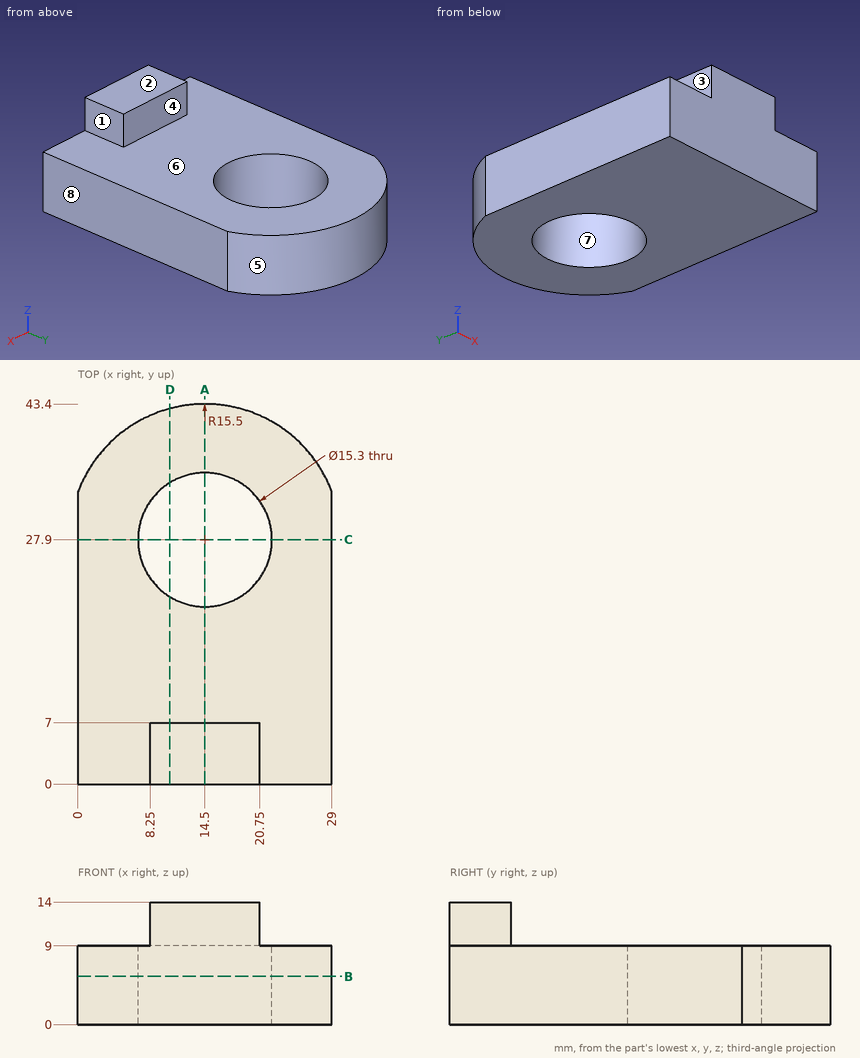
Design review of the part shown in the three views and the two pictorial views. Dimensions are in mm from the part's minimum x, y and z. A direction names the side the tool comes from. Round coordinates to 2 decimals unless told otherwise and drop trailing zeros. Write each loop counter-clockwise with the first axis right and the second up, starting at its lowest first coordinate (ties: lowest second). Pieces come first, ordered by that corner, then holes. Notation, with made-up numbers: (-28, 86.5) -> (18, 86.5) arc R28 cw to (18, 125.5) -> close; hole circle Ø10 at (84.5, 33). An arc over 180 degrees is marked (long way). One line per question, with ' | ' between items. Start each with the question number.
1) Add section D-D (x = 10.5). Write out the cut boundary in (y, z), and give its area (3 significant figures).
2) Mouldability with a two-part tool opening along X and no side actions: class the marked faces 6, 7 and 8 as +X half, -X half, draft (parallel to the pull), parting line (faces both ways), or undercut.
3) Add section C-C (y = 27.9). Write out the cut boundary in (x, z).
4) For pin 1 Ø8.5 at (x, y) = (19.5, 24.5) entering from +Z; pin 2 Ø5.5 at (x, z) = (17.5, 12) entering from +Y; pin 3 Ø1.5 at (y, z) = (3.5, 11.5) entering from -X, all flat-tipped, find the tip position at first contact; note any pin that passes through.
5) Add section A-A (x = 14.5). Write out the cut boundary in (y, z), and give its area (3 significant figures).
6) Add section B-B (z = 5.5). Write out the cut boundary in (x, y), and give its area (3 significant figures).
7) Machinability: for the marked faces 1, 2, 3, 4 and 5, which of the approach directions +Z, -Z, +X, -X, +Y, -Y give a long, thin tool a straight path to every point of the face, cutting with its end or side? Answer none if there is none.
8) Wall thickness on line 1 along Y through (x, z) = (14.5, 7.25); line 2 along Z through (x, y) = (24.25, 31); line 3 along Y through (x, z) = (14.75, 9.25): over which ranges is each line inside the solid? List them lowest first.
Reported:
1) outline: (0, 0) -> (21.38, 0) -> (21.38, 9) -> (7, 9) -> (7, 14) -> (0, 14) -> close; (34.42, 0) -> (42.87, 0) -> (42.87, 9) -> (34.42, 9) -> close | area: 303 mm²
2) face 6: draft | face 7: undercut | face 8: +X half
3) outline: (0, 0) -> (6.85, 0) -> (6.85, 9) -> (0, 9) -> close; (22.15, 0) -> (29, 0) -> (29, 9) -> (22.15, 9) -> close
4) pin 1: stops at z = 9 | pin 2: stops at y = 7 | pin 3: stops at x = 8.25
5) outline: (0, 0) -> (20.25, 0) -> (20.25, 9) -> (7, 9) -> (7, 14) -> (0, 14) -> close; (35.55, 0) -> (43.4, 0) -> (43.4, 9) -> (35.55, 9) -> close | area: 288 mm²
6) outline: (0, 0) -> (29, 0) -> (29, 33.38) arc R15.5 ccw to (0, 33.38) -> close; hole circle Ø15.3 at (14.5, 27.9) | area: 995 mm²
7) face 1: +Z, +X, +Y, -Y | face 2: +Z, +X, -X, +Y, -Y | face 3: +Z, -X, +Y, -Y | face 4: +Z, +X, -X, +Y | face 5: +Z, -Z, +Y
8) line 1: y = 0 to 20.25, 35.55 to 43.4 | line 2: z = 0 to 9 | line 3: y = 0 to 7
